Autodesk Inventor part; units mm, degrees
ref_plane "YZ Plane" through (0, 0, 0) normal (1, 0, 0) x (0, 1, 0)
ref_plane "XZ Plane" through (0, 0, 0) normal (0, 1, 0) x (-1, 0, 0)
ref_plane "XY Plane" through (0, 0, 0) normal (0, 0, 1) x (1, 0, 0)
sketch "Boceto1" plane through (0, 0, 0) normal (1, 0, 0) x (0, 1, 0)
  line L0 (1.5, 0) -> (1.5, -5)
  line L1 (1.5, -5) -> (4, -5)
  line L2 (4, -5) -> (4, -2)
  line L3 (4, -2) -> (10, -2)
  line L4 (10, -2) -> (10, 0)
  line L5 (10, 0) -> (1.5, 0)
  line L6 (0, 0) -> (0, -11.2963)
  line L7 (0, -13.5555) -> (0, 2.2593)
  dimension "d0" = 10
  dimension "d1" = 1.5
  dimension "d4" = 4
  dimension "d6" = 2
  dimension "d7" = 5
revolve "Revolución1" add sketch "Boceto1" angle 360 about axis through (0, 0, -10) along (0, 0, 1)
sketch "Boceto2" plane through (0, 0, -2) normal (0, 0, -1) x (-1, 0, 0)
  circle A0 centre (0, 7) radius 0.75
  circle A1 centre (-7, 0) radius 0.75
  circle A2 centre (0, -7) radius 0.75
  circle A3 centre (7, 0) radius 0.75
  circle A4 centre (0, 0) radius 7
  dimension "d25" = 14
  dimension "d20" = 1.5
  dimension "d23" = 360
extrude "Extrusión1" cut sketch "Boceto2" against normal through all contours A0 A4 | A4 A0 | A4 A1 | A1 A4 | A4 A3 | A3 A4 | A4 A2 | A2 A4
properties part number "Brida de servo"
The listing builds one solid part. Answer for the finished solid, in the listing's coordinates (mm). Coordinates: 2 decimals unless noted, no trailing zeros. Write each loop counter-clockwise with the first axis right and the second up, starting at its lowest first coordinate (ties: lowest second). Pieces come first, ordered by that corner, then holes. Notation, with made-up numbers: (-28, 55) - (9, 55) arc R14 cw to (9, 60) - close; hole circle Ø1 at (-35, 5). An arc over 180 degrees is marked (long way). Return JSON: item names as keys, results as strings. Group by question number.
Q1. For a pull along X with two mould halves and no side action, classify faces 1 (the cylindrical face through (0.163, 6.268, -1.014)), 2 (the cylindrical face through (3.905, -0.867, -3.479)), 3 (the flat face through (-0.1, 4.3, -2)), 4 (the cylindrical face through (7.75, 0.03, -1.01)) as +X half, -X half, draft (parallel to the pull), parting line (faces both ways), or undercut.
Q2. The part is cut by section C-C on y = 7. Write down the section's boundary in (x, z), and give its area (3 significant figures).
Q3. The part is cut by section A-A on x = 0. Write down the section's boundary in (y, z).
Q4. Find the intervals of material crossed by line 1 along X through (y, z) = (0, -1.45); line 2 along X through (y, z) = (0, -3.8), in increasing order. Write a range as [from, to].
Q5. Flat-ended cylindrical pins translate along their axes: pin 1 Ø2 at (x, z) = (0.5, -1.5) entering from +Y; pin 2 Ø2 at (x, y) = (0, -7) entering from -Z. Find the tip coordinate at first contact, or state that the pin passes through.
Q6. The part is cut by section B-B on z = -1.05. Write down the section's boundary in (x, y).
Evaluation:
{
 "1": {"face 1": "undercut", "face 2": "parting line", "face 3": "draft", "face 4": "undercut"},
 "2": {"outline": "(-7.14, -2) - (-0.75, -2) - (-0.75, 0) - (-7.14, 0) - close; (0.75, -2) - (7.14, -2) - (7.14, 0) - (0.75, 0) - close", "area": "25.6 mm2"},
 "3": {"outline": "(-10, -2) - (-7.75, -2) - (-7.75, 0) - (-10, 0) - close; (-6.25, -2) - (-4, -2) - (-4, -5) - (-1.5, -5) - (-1.5, 0) - (-6.25, 0) - close; (1.5, -5) - (4, -5) - (4, -2) - (6.25, -2) - (6.25, 0) - (1.5, 0) - close; (7.75, -2) - (10, -2) - (10, 0) - (7.75, 0) - close"},
 "4": {"line 1": "x = [-10, -7.75], [-6.25, -1.5], [1.5, 6.25], [7.75, 10]", "line 2": "x = [-4, -1.5], [1.5, 4]"},
 "5": {"pin 1": "stops at y = 10", "pin 2": "stops at z = -2"},
 "6": {"outline": "circle Ø20 at (0, 0); hole circle Ø1.5 at (-7, 0); hole circle Ø3 at (0, 0); hole circle Ø1.5 at (0, -7); hole circle Ø1.5 at (0, 7); hole circle Ø1.5 at (7, 0)"}
}
